Verification items for the finished model (mm, model axes). A direction names the side the tool comes from. Coordinates: 2 decimals unless noted, no trailing zeros. Loops run counter-clockwise (first coordinate to the right, second up) from the corner with the lowest first, then second, coordinate; pieces in that order, holes last.
Q1. Sectioned sample at B-B (y = 7.75). Enter the section's corners in (x, z) (1 decimal), then the cut area to 3 significant figures.
Q2. Material ranges on probe 1 along X at (y, z) = (13.5, 0); probe 2 along X at (y, z) = (8, 0); probe 3 along Y at (x, z) = (-1.5, -4.5), recorded low to high.
Q3. Mould release check, pull along X, two halves, no side actions. Record for faces 5 (the face through (7.662, 14.451, -0.595)), 6 (the face through (-1.39, 14.45, -6.54)), 7 (the face through (-6.686, 14.451, 0.703)): +X half, -X half, draft (parallel to the pull), parting line (faces both ways), or undercut.
Q4. Sectioned sample at C-C (x = 9.75). Enter the section's corners in (y, z), then the cut area to 3 significant figures.
Q5. Go/stop test with flat-tipped pins: P1, Ø5, axis at y = 9, z = -7.5, coming from the +X side; P2, Ø8, axis at x = 0, z = 0, coming from the +Y side; P3, Ø1.3, axis at y = 15.5, z = 6.5, coming from the +X side; P4, Ø1.5, axis at x = 4.5, y = 14.5, coming from the +Z side. Record where each tip stops, or that it passes through.
Q6. Access from +Z, -Z, +X, -X, +Y, -Y to the whole of each face (thin tool, end or side, straight path). Record for faces 1 (the face through (-4.346, 14.451, -6.338)), 2 (the face through (5.59, 14.45, -5.32)), 3 (the face through (-5.58, 14.451, 2.494)), 4 (the face through (1.39, 14.45, -6.54)).
Q7. Sectioned sample at A-A (x = -2). Enter the section's corners in (y, z), then the cut area to 3 significant figures.
```python
from build123d import *

# Parameters (mm, degrees)
SKETCH1_R           = 11.1125
BOSS_EXTRUDE1_DEPTH = 18
CUT_EXTRUDE2_START  = -7
CUT_EXTRUDE2_DEPTH  = 7
CIRPATTERN1_COUNT   = 15
SKETCH3_R           = 6.5
CUT_EXTRUDE3_DEPTH  = 3
SKETCH4_R           = 4.5
CUT_EXTRUDE4_DEPTH  = 22.724992808


with BuildPart() as part:
    # Sketch1 → Boss-Extrude1 (new body)
    with BuildSketch(Plane(origin=(0, 0, 0), x_dir=(1, 0, 0), z_dir=(0, 1, 0))):
        with Locations(Location((0, 0, 0), (0, 0, 270))):
            Circle(SKETCH1_R)
    extrude(amount=BOSS_EXTRUDE1_DEPTH)

    # Sketch2 → Cut-Extrude2 (cut)
    with BuildSketch(Plane(origin=(0, 18, 0), x_dir=(1, 0, 0), z_dir=(0, 1, 0)).offset(CUT_EXTRUDE2_START)):
        with BuildLine():
            Line((10.151773898, 4.519860946), (7.411137525, 3.299651017))
            ThreePointArc((7.411137525, 3.299651017), (7.494972707, 3.104519345), (7.57367121, 2.907259991))
            Line((7.57367121, 2.907259991), (6.959086209, 2.261144177))
            Line((6.959086209, 2.261144177), (5.813332956, 1.888866378))
            ThreePointArc((5.813332956, 1.888866378), (5.978927209, 1.27086021), (6.079015085, 0.638930232))
            Line((6.079015085, 0.638930232), (7.234212217, 0.760346343))
            Line((7.234212217, 0.760346343), (8.101382101, 0.424575445))
            ThreePointArc((8.101382101, 0.424575445), (8.109720049, 0.212360493), (8.1125, 0))
            Line((8.1125, 0), (11.1125, 0))
            ThreePointArc((11.1125, 0), (10.869665213, 2.310418664), (10.151773898, 4.519860946))
        make_face()
    cut_extrude2 = extrude(amount=CUT_EXTRUDE2_DEPTH, mode=Mode.SUBTRACT)

    # CirPattern1: Cut-Extrude2 ×15 about axis
    cirpattern1_axis = Axis((0, 0, 0), (0, 1, 0))
    for i in range(1, CIRPATTERN1_COUNT):
        add(cut_extrude2.rotate(cirpattern1_axis, i * 360 / CIRPATTERN1_COUNT), mode=Mode.SUBTRACT)

    # Sketch3 → Cut-Extrude3 (cut)
    with BuildSketch(Plane.XZ):
        with Locations(Location((0, 0, 0), (0, 0, 270))):
            Circle(SKETCH3_R)
    extrude(amount=-CUT_EXTRUDE3_DEPTH, mode=Mode.SUBTRACT)

    # Sketch4 → Cut-Extrude4 (cut, through all)
    with BuildSketch(Plane.XZ.offset(-3)):
        with Locations(Location((0, 0, 0), (0, 0, 270))):
            Circle(SKETCH4_R)
    extrude(amount=-CUT_EXTRUDE4_DEPTH, mode=Mode.SUBTRACT)


solid = part.part
```
Geometry check:
1. outline: circle Ø22.2 at (0, 0); hole circle Ø9 at (0, 0)
1. area: 324 mm2
2. probe 1: x = -6.11 to -4.5, 4.5 to 8.11
2. probe 2: x = -11.11 to -4.5, 4.5 to 11.11
2. probe 3: y = 3 to 18
3. face 5: +X half
3. face 6: undercut
3. face 7: -X half
4. outline: (0, -5.33) - (11, -5.33) - (11, 5.33) - (0, 5.33) - close
4. area: 117 mm2
5. P1: stops at x = 9.92
5. P2: passes through
5. P3: stops at x = 5.62
5. P4: stops at z = 6.3
6. face 1: -X, +Y
6. face 2: +X, +Y
6. face 3: +Y
6. face 4: -Z, +Y
7. outline: (0, -10.93) - (11, -10.93) - (11, -5.78) - (18, -5.78) - (18, -4.03) - (3, -4.03) - (3, -6.18) - (0, -6.18) - close; (0, 6.18) - (3, 6.18) - (3, 4.03) - (18, 4.03) - (18, 5.78) - (11, 5.78) - (11, 10.93) - (0, 10.93) - close
7. area: 163 mm2
